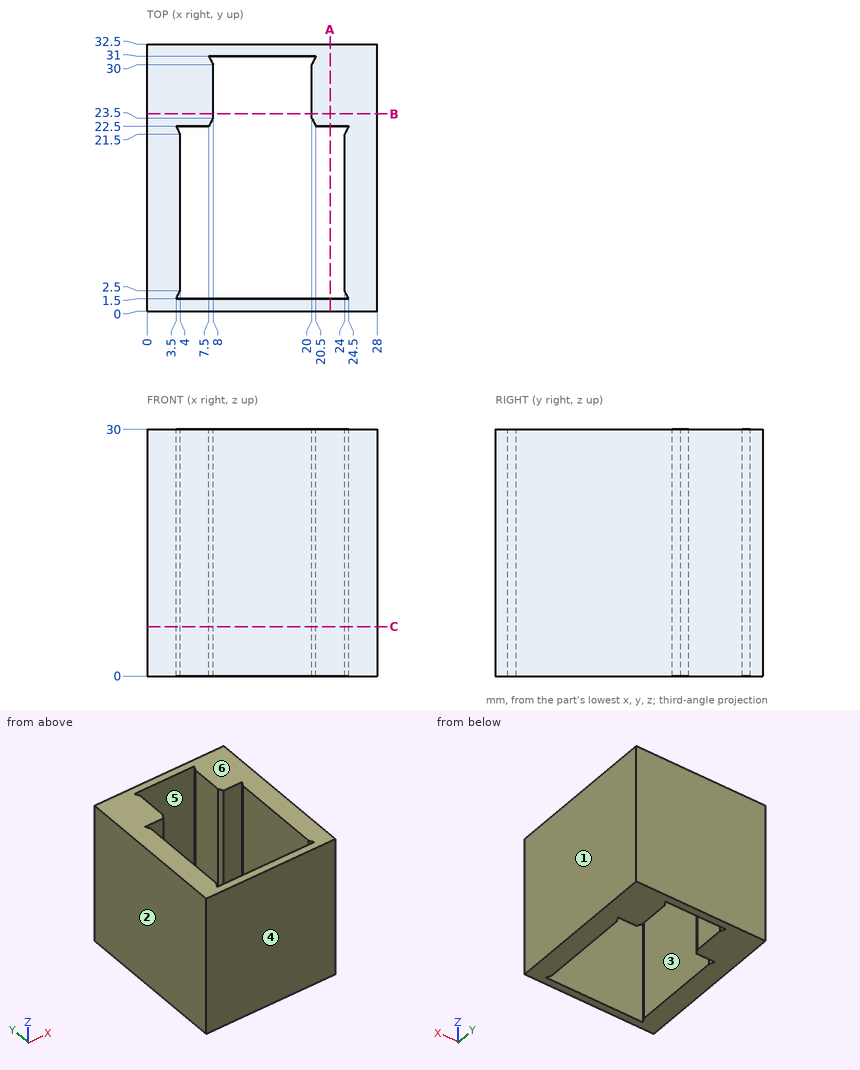
Study the drawing (mm; zero at the part's minimum x, y, z) and answer. A direction names the side the tool comes from. Give positions to 0.01 mm unless a question says otherwise; leave off trailing zeros. Loops run counter-clockwise (first coordinate to the right, second up) from the corner with the lowest first, then second, coordinate; pieces in that order, holes last. Notation, with made-up numbers: (72, 47) -> (127, 47) arc R10 ccw to (127, 55) -> close; hole circle Ø10 at (-22, 59). An arc over 180 degrees is marked (long way). Use a Markdown table: item, result. Add a question column.
1) The part is cut by section C-C, the plane z = 6. Determine the outline of the cut face in (x, y), plus the area to 3 significant figures.
2) Which of the six approach directions +Z, -Z, +X, -X, +Y, -Y give full straight-line access (tool end or side, diameter ignored) to the marked faces 5 and 6?
3) The part is cut by section A-A, the plane x = 22.25. Determine the outline of the cut face in (y, z), plus the area to 3 significant figures.
4) Each of these flat-tipped pins is pushed along its axis until it touches: P1, Ø4, axis at y = 14, z = 19, coming from the -X side; P2, Ø10, axis at x = 14.5, y = 12, coming from the +Z side. Where does it stop, or does it pass through?
5) The part is cut by section B-B, the plane y = 24. Determine the outline of the cut face in (x, z).
6) Consider line 1 along Y through (x, z) = (6.5, 13); line 2 along X through (y, z) = (9, 9); line 3 along Y through (x, z) = (17, 17.5). Determine where each line is inside the solid, lowest interval first.
7) For a pull along X with two mould halves and no side action, classify the marked faces 1, 2, 3 and 4 as +X half, -X half, draft (parallel to the pull), parting line (faces both ways), or undercut.
Reported:
| question | item | result |
|---|---|---|
| 1 | outline | (0, 0) -> (28, 0) -> (28, 32.5) -> (0, 32.5) -> close; hole (3.5, 1.5) -> (24.5, 1.5) -> (24, 2.5) -> (24, 21.5) -> (24.5, 22.5) -> (20.5, 22.5) -> (20, 23.5) -> (20, 30) -> (20.5, 31) -> (7.5, 31) -> (8, 30) -> (8, 23.5) -> (7.5, 22.5) -> (3.5, 22.5) -> (4, 21.5) -> (4, 2.5) -> close |
| 1 | area | 386 mm^2 |
| 2 | face 5 | +Z, -Z |
| 2 | face 6 | +Z, +X, -X, +Y, -Y |
| 3 | outline | (0, 0) -> (1.5, 0) -> (1.5, 30) -> (0, 30) -> close; (22.5, 0) -> (32.5, 0) -> (32.5, 30) -> (22.5, 30) -> close |
| 3 | area | 345 mm^2 |
| 4 | P1 | stops at x = 0 |
| 4 | P2 | passes through |
| 5 | outline | (0, 0) -> (8, 0) -> (8, 30) -> (0, 30) -> close; (20, 0) -> (28, 0) -> (28, 30) -> (20, 30) -> close |
| 6 | line 1 | y = 0 to 1.5, 22.5 to 32.5 |
| 6 | line 2 | x = 0 to 4, 24 to 28 |
| 6 | line 3 | y = 0 to 1.5, 31 to 32.5 |
| 7 | face 1 | +X half |
| 7 | face 2 | -X half |
| 7 | face 3 | undercut |
| 7 | face 4 | draft |
